Geometry: final body of the model. Coordinates: model frame, mm. Give positions to 0.01 mm unless a question says otherwise; leave off trailing zeros. Order: outer loops, then holes, each group sorted by start corner. A loop starts at its lowest first (then second) coordinate and runs counter-clockwise, first axis right, second up. Notation, with made-up numbers: (-0.5, 39.25) -> (52.5, 39.25) arc R25 cw to (52.5, 78.25) -> close; hole circle Ø2 at (-5, 46.5). An arc over 180 degrees is marked (long way). Write item = value, one per line.
```python
from build123d import *

# Parameters (mm, degrees)
BOX005_W          = 71
BOX005_H          = 76
BOX005_DEPTH      = 2
FILLET003002012_R = 20
FILLET003002013_R = 30
FILLET003002014_R = 30
FILLET003002015_R = 30


with BuildPart() as part:
    # Box005 → Box005 (new body)
    with BuildSketch(Plane(origin=(-35.5, -38, 20), x_dir=(1, 0, 0), z_dir=(0, 0, 1))):
        with Locations((35.5, 38)):
            Rectangle(BOX005_W, BOX005_H)
    extrude(amount=BOX005_DEPTH)

    # Fillet003002012
    fillet003002012_edges = [part.edges().sort_by_distance(p)[0] for p in [
        (-35.5, -38, 21),
    ]]
    fillet(fillet003002012_edges, radius=FILLET003002012_R)

    # Fillet003002013
    fillet003002013_edges = [part.edges().sort_by_distance(p)[0] for p in [
        (-35.5, 38, 21),
    ]]
    fillet(fillet003002013_edges, radius=FILLET003002013_R)

    # Fillet003002014
    fillet003002014_edges = [part.edges().sort_by_distance(p)[0] for p in [
        (35.5, 38, 21),
    ]]
    fillet(fillet003002014_edges, radius=FILLET003002014_R)

    # Fillet003002015
    fillet003002015_edges = [part.edges().sort_by_distance(p)[0] for p in [
        (35.5, -38, 21),
    ]]
    fillet(fillet003002015_edges, radius=FILLET003002015_R)


solid = part.part
```
1) Section query B-B (x = -19). Output: boundary loops of the cut face in (y, z).
Check sheet entries:
outline = (-37.69, 20) -> (34.79, 20) -> (34.79, 22) -> (-37.69, 22) -> close
2) Line query: line 1 (X direction, y = -23, z = 21.2); line 2 (Y direction, x = 7, z = 21.25); line 3 (Y direction, x = -19, z = 20.4). Output: solid intervals per line, ascending. Write a range as from..to.
Check sheet entries:
line_1 = -34.86..31.48
line_2 = -37.96..37.96
line_3 = -37.69..34.79
3) Section query C-C (y = -20.5). Output: boundary loops of the cut face in (x, z).
Check sheet entries:
outline = (-35.34, 20) -> (32.77, 20) -> (32.77, 22) -> (-35.34, 22) -> close
4) Section query A-A (z = 21.3). Output: boundary loops of the cut face in (x, y), plus the area to 3 significant figures.
Check sheet entries:
outline = (-35.5, -18) arc R20 ccw to (-15.5, -38) -> (5.5, -38) arc R30 ccw to (35.5, -8) -> (35.5, 8) arc R30 ccw to (5.5, 38) -> (-5.5, 38) arc R30 ccw to (-35.5, 8) -> close
area = 4,730 mm²
